Drawing for the job (mm, zero at the part's lowest x, y, z). A direction names the side the tool comes from. Give positions to 0.01 mm unless a question says otherwise; leave off trailing zeros. Write each loop counter-clockwise with the first axis right and the second up, starting at its lowest first coordinate (ties: lowest second). Pieces come first, ordered by that corner, then holes.
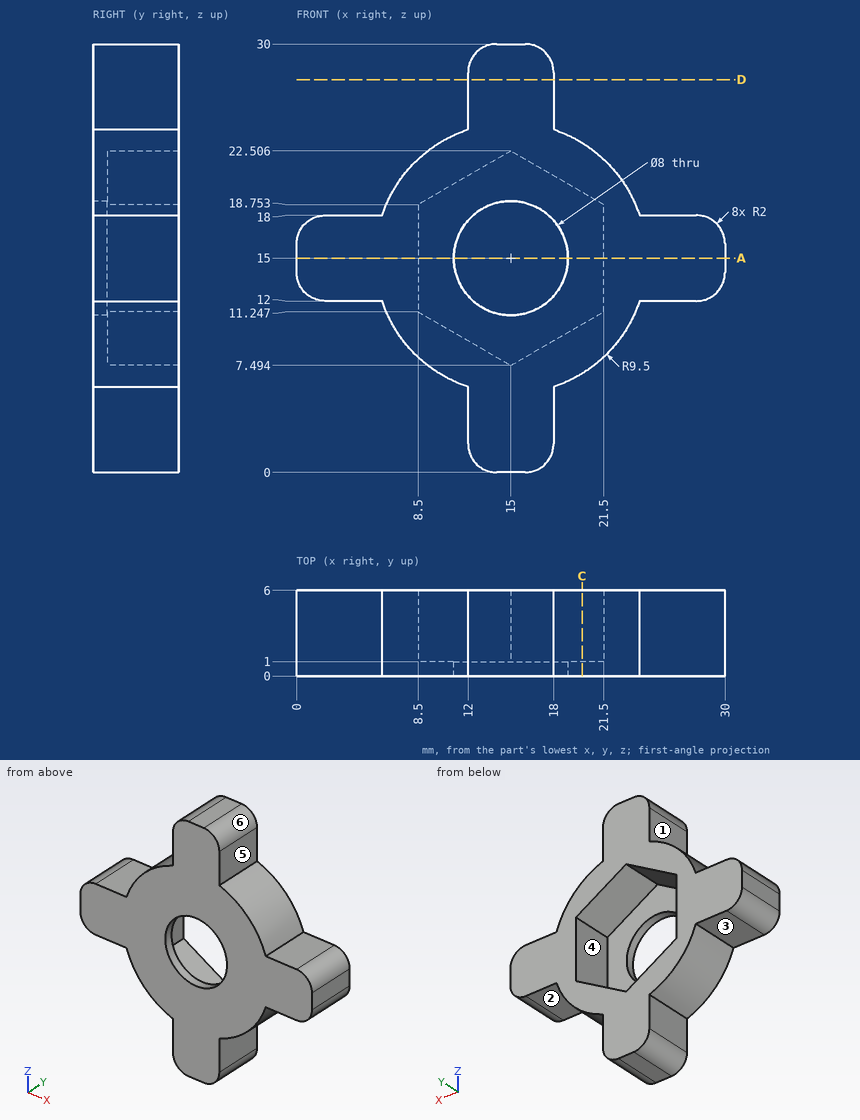
1. Pull direction Z, two halves, no side cores. Call the marked faces 4, 5 and 6: +Z half, -Z half, draft (parallel to the pull), parting line (faces both ways), or undercut.
Calculated:
face 4: undercut
face 5: draft
face 6: +Z half
2. Slice it at A-A, the plane z = 15. Write the cut outline in (x, y), and give its area (3 significant figures).
Calculated:
outline: (0, 0) - (11, 0) - (11, 1) - (8.5, 1) - (8.5, 6) - (0, 6) - close; (19, 0) - (30, 0) - (30, 6) - (21.5, 6) - (21.5, 1) - (19, 1) - close
area: 107 mm2
3. Probe probe 1 along X at (y, z) = (0.4, 15); probe 2 along X at (y, z) = (4.7, 26.75). List the from-to ranges inside material, lowest first.
Calculated:
probe 1: x = 0 to 11, 19 to 30
probe 2: x = 12 to 18
4. Pin check, flat tips, straight feed: P1, Ø2, axis at x = 3.5, y = 4, coming from the -Z side; P2, Ø1.2, axis at x = 25.5, y = 4, coming from the +Z side; P3, Ø3, axis at y = 2.5, z = 3, coming from the +X side. Stop position of each tip, or through.
Calculated:
P1: stops at z = 12
P2: stops at z = 18
P3: stops at x = 18
5. Slice it at C-C, the plane x = 20. Write the cut outline in (y, z).
Calculated:
outline: (0, 6.92) - (6, 6.92) - (6, 10.38) - (1, 10.38) - (1, 19.62) - (6, 19.62) - (6, 23.08) - (0, 23.08) - close
6. Which spindle directions (+Z, -Z, +X, -X, +Y, -Y) get a long thin tool onto all of the face, cutting with end or side? Do the marked faces 1, 2 and 3. Say none if no direction does.
Calculated:
face 1: +Z, -X, +Y, -Y
face 2: -Z, +X, +Y, -Y
face 3: -Z, -X, +Y, -Y
7. Slice it at D-D, the plane z = 27.5. Write the cut outline in (x, y), and give its area (3 significant figures).
Calculated:
outline: (12, 0) - (18, 0) - (18, 6) - (12, 6) - close
area: 36.0 mm2
